```python
from build123d import *

# Parameters (mm, degrees)
F0_W     = 6.35
F0_H     = 6.35
F1_DEPTH = 6.35
F2_SIZE  = 1.016
F3_SIZE  = 1.016


with BuildPart() as f1:
    # F0 (on Front) → F1 (new body)
    with BuildSketch(Plane.XZ):
        Polygon((0, -12.7), (6.35, -12.7), (6.35, 0), (12.7, 0), (12.7, 6.35), (6.35, 6.35), (0, 6.35), (-12.7, 6.35), (-12.7, -12.7), (-6.35, -12.7), (-6.35, -6.35), (0, -6.35), align=None)
        with Locations((3.175, 9.525)):
            Rectangle(F0_W, F0_H)
    extrude(amount=F1_DEPTH)

    # F2
    f2_edges = [f1.edges().sort_by_distance(p)[0] for p in [
        (-12.7, -6.35, -3.175),
    ]]
    chamfer(f2_edges, length=F2_SIZE)

    # F3
    f3_edges = [f1.edges().sort_by_distance(p)[0] for p in [
        (3.175, -6.35, 12.7),
    ]]
    chamfer(f3_edges, length=F3_SIZE)


solid = f1.part
```
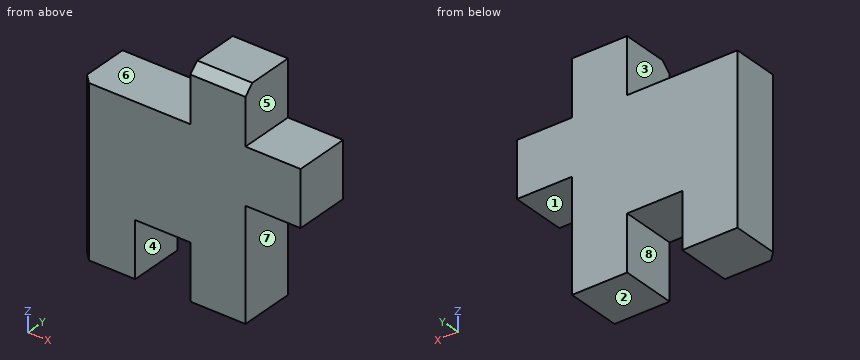
Source: CAD feature listing. Evaluate the final solid. Frame: model axes, mm. Face numbers are marked on the shaded views. A direction names the side the tool comes from. Round coordinates to 2 decimals unless told otherwise and drop trailing zeros. Loops run counter-clockwise (first coordinate to the right, second up) from the corner with the lowest first, then second, coordinate; pieces in that order, holes last. Notation, with made-up numbers: M 3.25,69.5 L 51.25,69.5 A34 ccw 51.25,104.5 Z; hole C -30.75,46 d11. An arc over 180 degrees is marked long. Use a Markdown table: item, result. Add a question column.
1. Cut plane C-C, the plane z = -2. Output: boundary loops of the cut face in (x, y), and give its area (3 significant figures).
2. Ray query, line 1 along X through (y, z) = (-4.25, -6.5); line 2 along X through (y, z) = (-2.5, 6.5); line 3 along X through (y, z) = (-2.5, -1.25). Return the intervals inside material, ascending. Write a range as [from, to].
3. Contact query for flat-ended pins moving along their axis: pin 1 (3 mm diameter, centred on y = -3.5, z = -10, fed in from +X); pin 2 (1.9 mm diameter, centred on x = 11, y = -3, fed in from -Z); pin 3 (1.9 mm diameter, centred on x = 11, y = -3.5, fed in from +Z); pin 4 (2 mm diameter, centred on x = -6, z = -1.5, fed in from +Y). Output: stop coordinate, or through.
4. Pull-direction query (X, two-part tool) for the marked faces 6, 7 and 8; classes: +X half, -X half, draft (parallel to the pull), parting line (faces both ways), or undercut.
5. Cut plane A-A, the plane z = -8.25. Output: boundary loops of the cut face in (x, y).
6. Cut plane B-B, the plane y = -1.75. Output: boundary loops of the cut face in (x, z).
7. Cut plane D-D, the plane x = -6. Output: boundary loops of the cut face in (y, z), and give its area (3 significant figures).
8. Set-up query: the marked faces 1, 2, 3, 4 and 5. Return all of +Z, -Z, +X, -X, +Y, -Y with unobstructed straight access to the full face (end or side cutting, diameter ignored); none if empty.
Solution:
| question | item | result |
|---|---|---|
| 1 | outline | M -12.7,-5.33 L -11.68,-6.35 L 6.35,-6.35 L 6.35,0 L -12.7,0 Z |
| 1 | area | 120 mm2 |
| 2 | line 1 | x = [-12.7, -6.35], [0, 6.35] |
| 2 | line 2 | x = [0, 6.35] |
| 2 | line 3 | x = [-12.7, 6.35] |
| 3 | pin 1 | stops at x = 6.35 |
| 3 | pin 2 | stops at z = 0 |
| 3 | pin 3 | stops at z = 6.35 |
| 3 | pin 4 | stops at y = 0 |
| 4 | face 6 | draft |
| 4 | face 7 | +X half |
| 4 | face 8 | undercut |
| 5 | outline | M -12.7,-5.33 L -11.68,-6.35 L -6.35,-6.35 L -6.35,0 L -12.7,0 Z; M 0,-6.35 L 6.35,-6.35 L 6.35,0 L 0,0 Z |
| 6 | outline | M -12.7,-12.7 L -6.35,-12.7 L -6.35,-6.35 L 0,-6.35 L 0,-12.7 L 6.35,-12.7 L 6.35,0 L 12.7,0 L 12.7,6.35 L 6.35,6.35 L 6.35,12.7 L 0,12.7 L 0,6.35 L -12.7,6.35 Z |
| 7 | outline | M -6.35,-6.35 L 0,-6.35 L 0,6.35 L -6.35,6.35 Z |
| 7 | area | 80.6 mm2 |
| 8 | face 1 | -Z, +X, +Y, -Y |
| 8 | face 2 | -Z, +X, -X, +Y, -Y |
| 8 | face 3 | +Z, -X, +Y, -Y |
| 8 | face 4 | -Z, +Y, -Y |
| 8 | face 5 | +Z, +X, +Y, -Y |
